Part model, mm, in its own coordinate system. A direction names the side the tool comes from. Coordinates: 2 decimals unless noted, no trailing zeros. Loops run counter-clockwise (first coordinate to the right, second up) from the corner with the lowest first, then second, coordinate; pieces in that order, holes last. Notation, with made-up numbers: (87.25, 49) - (145.25, 49) arc R29 cw to (145.25, 87) - close; hole circle Ø1 at (-16.5, 44). An arc over 180 degrees is marked (long way). Use a Markdown table: item, result. Add a question column.
1. Pull direction Z, two halves, no side cores. Call faces 6 (the flat face through (13, 2, 0)), 7 (the flat face through (-6, 34, -1.75)), 8 (the flat face through (-6, 34, 1.75)): pulls with the +Z half, pulls with the -Z half, needs draft (parallel to the pull), parting line crosses it, or undercut.
2. Band-saw the part on D-D, the plane x = 3.5. Give the cut face in (y, z), plus the area to 3 significant figures.
3. Drop flat-ended pins along their axis: pin 1 (2.5 mm diameter, centred on y = 10.45, z = -8, fed in from -X); pin 2 (2 mm diameter, centred on x = -6, y = 35, fed in from +Z); pin 3 (3.5 mm diameter, centred on x = -7, y = 34.5, fed in from -Z); pin 4 (4 mm diameter, centred on x = 27, y = 25.5, fed in from -Z). Give the stop position or say it passes through.
4. Band-saw the part on B-B, the plane y = 41.95. Give the cut face in (x, z).
5. Band-saw the part on A-A, the plane z = 0. Give the cut face in (x, y).
6. 3-axis set-ups, long thin cutter, end or side, ignore diameter. For faces 1 (the cylindrical face through (6.31, 42.54, 9.29)), 2 (the flat face through (5.5, 10, -8)), 3 (the flat face through (4, 42, -6.5)), 4 (the cylindrical face through (38.78, 15.12, 10.15)), 5 (the flat face through (14, 5, 0)): which of +Z, -Z, +X, -X, +Y, -Y reach the whole face in a straight line?
7. Band-saw the part on C-C, the plane z = -8. Give the cut face in (x, y).
8. Wall check: probe 1 along Z at (x, y) = (3, 10); probe 2 along Y at (x, z) = (4.45, 9.2); probe 3 along Y at (x, z) = (4.45, -8.35). Give the ranges that are in metal, low to high. Write a range as [from, to].
from build123d import *

# Parameters (mm, degrees)
SKETCH1_W               = 23
SKETCH1_H               = 46.4
BOSS_EXTRUDE1_DEPTH     = 12
SKETCH6_R               = 1.95
CUT_EXTRUDE1_DEPTH      = 5.5
SKETCH7_R               = 2.7
BOSS_EXTRUDE2_DEPTH     = 9
SKETCH8_W               = 7
SKETCH8_H               = 0.95
CUT_EXTRUDE2_DEPTH      = 47.4
SKETCH9_R               = 1.95
CUT_EXTRUDE3_DEPTH      = 5.5
SKETCH10_R              = 10.15
BOSS_EXTRUDE3_DEPTH     = 32
SKETCH11_W              = 32
SKETCH11_H              = 2.45
CUT_EXTRUDE4_DEPTH      = 13
CUT_EXTRUDE4_DEPTH_BACK = 13
SKETCH12_W              = 3
SKETCH12_H              = 9
CUT_EXTRUDE5_DEPTH      = 5


with BuildPart() as part:
    # Sketch1 → Boss-Extrude1 (new body, symmetric)
    with BuildSketch(Plane.XY):
        with Locations((11.5, 23.2)):
            Rectangle(SKETCH1_W, SKETCH1_H)
    extrude(amount=BOSS_EXTRUDE1_DEPTH, both=True)

    # Sketch6 → Cut-Extrude1 (cut)
    with BuildSketch(Plane.XY.offset(12)):
        with Locations((4.45, 41.95)):
            Circle(SKETCH6_R)
        with Locations((4.45, 25.95)):
            Circle(SKETCH6_R)
    cut_extrude1 = extrude(amount=-CUT_EXTRUDE1_DEPTH, mode=Mode.SUBTRACT)

    # Mirror1: Cut-Extrude1 across plane
    add(cut_extrude1.mirror(Plane.XY), mode=Mode.SUBTRACT)

    # Sketch7 → Boss-Extrude2 (add)
    with BuildSketch(Plane.ZY):
        with Locations((0, 34.2)):
            Circle(SKETCH7_R)
    extrude(amount=BOSS_EXTRUDE2_DEPTH)

    # Sketch8 → Cut-Extrude2 (cut, through all)
    with BuildSketch(Plane(origin=(0, 0, 0), x_dir=(1, 0, 0), z_dir=(0, 1, 0))):
        with Locations((-5.5, 2.225)):
            Rectangle(SKETCH8_W, SKETCH8_H)
        with Locations((-5.5, -2.225)):
            Rectangle(SKETCH8_W, SKETCH8_H)
    extrude(amount=CUT_EXTRUDE2_DEPTH, mode=Mode.SUBTRACT)

    # Sketch9 → Cut-Extrude3 (cut)
    with BuildSketch(Plane.ZY):
        with Locations((-8, 10.45)):
            Circle(SKETCH9_R)
        with Locations((8, 10.45)):
            Circle(SKETCH9_R)
    extrude(amount=-CUT_EXTRUDE3_DEPTH, mode=Mode.SUBTRACT)

    # Sketch10 → Boss-Extrude3 (add)
    with BuildSketch(Plane(origin=(23, 0, 0), x_dir=(0, 0, -1), z_dir=(1, 0, 0))):
        with Locations((0, 15)):
            Circle(SKETCH10_R)
    extrude(amount=BOSS_EXTRUDE3_DEPTH)

    # Sketch11 → Cut-Extrude4 (cut, two sides)
    with BuildSketch(Plane.XY) as cut_extrude4_sk:
        with Locations((39, 23.925)):
            Rectangle(SKETCH11_W, SKETCH11_H)
        with Locations((39, 6.075)):
            Rectangle(SKETCH11_W, SKETCH11_H)
    extrude(amount=CUT_EXTRUDE4_DEPTH, mode=Mode.SUBTRACT)
    extrude(cut_extrude4_sk.sketch, amount=-CUT_EXTRUDE4_DEPTH_BACK, mode=Mode.SUBTRACT)

    # Sketch12 → Cut-Extrude5 (cut)
    with BuildSketch(Plane.XZ):
        with Locations((14.5, 0)):
            Rectangle(SKETCH12_W, SKETCH12_H)
    extrude(amount=-CUT_EXTRUDE5_DEPTH, mode=Mode.SUBTRACT)


solid = part.part
Geometry check:
| question | item | result |
|---|---|---|
| 1 | face 6 | undercut |
| 1 | face 7 | pulls with the -Z half |
| 1 | face 8 | pulls with the +Z half |
| 2 | outline | (0, -12) - (24.25, -12) - (24.25, -6.5) - (27.65, -6.5) - (27.65, -12) - (40.25, -12) - (40.25, -6.5) - (43.65, -6.5) - (43.65, -12) - (46.4, -12) - (46.4, 12) - (43.65, 12) - (43.65, 6.5) - (40.25, 6.5) - (40.25, 12) - (27.65, 12) - (27.65, 6.5) - (24.25, 6.5) - (24.25, 12) - (0, 12) - close; hole circle Ø3.9 at (10.45, -8); hole circle Ø3.9 at (10.45, 8) |
| 2 | area | 1,010 mm^2 |
| 3 | pin 1 | stops at x = 5.5 |
| 3 | pin 2 | stops at z = 1.75 |
| 3 | pin 3 | stops at z = -1.75 |
| 3 | pin 4 | passes through |
| 4 | outline | (0, -12) - (2.5, -12) - (2.5, -6.5) - (6.4, -6.5) - (6.4, -12) - (23, -12) - (23, 12) - (6.4, 12) - (6.4, 6.5) - (2.5, 6.5) - (2.5, 12) - (0, 12) - close |
| 5 | outline | (-9, 31.5) - (0, 31.5) - (0, 0) - (13, 0) - (13, 5) - (16, 5) - (16, 0) - (23, 0) - (23, 7.3) - (55, 7.3) - (55, 22.7) - (23, 22.7) - (23, 46.4) - (0, 46.4) - (0, 36.9) - (-9, 36.9) - close |
| 6 | face 1 | +Z |
| 6 | face 2 | -X |
| 6 | face 3 | -Z |
| 6 | face 4 | +Z, +X |
| 6 | face 5 | -Y |
| 7 | outline | (0, 0) - (23, 0) - (23, 8.75) - (55, 8.75) - (55, 21.25) - (23, 21.25) - (23, 46.4) - (0, 46.4) - (0, 12.4) - (5.5, 12.4) - (5.5, 8.5) - (0, 8.5) - close; hole circle Ø3.9 at (4.45, 25.95); hole circle Ø3.9 at (4.45, 41.95) |
| 8 | probe 1 | z = [-12, -9.9], [-6.1, 6.1], [9.9, 12] |
| 8 | probe 2 | y = [0, 8.91], [11.99, 24], [27.9, 40], [43.9, 46.4] |
| 8 | probe 3 | y = [0, 8.53], [12.37, 24], [27.9, 40], [43.9, 46.4] |
